```python
from build123d import *

# Parameters (mm, degrees)
BOSS_EXTRUDE1_DEPTH = 1.5
SKETCH3_W           = 6.5
SKETCH3_H           = 6.5
CUT_EXTRUDE1_DEPTH  = 2


with BuildPart() as part:
    # Sketch2 → Boss-Extrude1 (new body)
    with BuildSketch(Plane.XY):
        with BuildLine():
            Line((-7.517156851, 8.129598801), (22.482843149, 8.129598801))
            Line((22.482843149, 8.129598801), (22.482843149, -7.870401199))
            Line((22.482843149, -7.870401199), (12.482843149, -7.870401199))
            ThreePointArc((12.482843149, -7.870401199), (5.615628068, -3.288438903), (-2.517156851, -1.870401199))
            Line((-2.517156851, -1.870401199), (-7.517156851, -1.870401199))
            Line((-7.517156851, -1.870401199), (-7.517156851, 8.129598801))
        make_face()
    extrude(amount=BOSS_EXTRUDE1_DEPTH)

    # Sketch3 → Cut-Extrude1 (cut)
    with BuildSketch(Plane.XY.offset(1.5)):
        with Locations((16.232843149, -1.120401199)):
            Rectangle(SKETCH3_W, SKETCH3_H)
    extrude(amount=-CUT_EXTRUDE1_DEPTH, mode=Mode.SUBTRACT)


solid = part.part
```
Here's how the part is built. I have some questions about the finished solid (model axes, mm). A direction names the side the tool comes from. Give positions to 0.01 mm unless a question says otherwise; leave off trailing zeros. Write each loop counter-clockwise with the first axis right and the second up, starting at its lowest first coordinate (ties: lowest second). Pieces come first, ordered by that corner, then holes. Notation, with made-up numbers: M 31.5,80 L 72.5,80 A17 cw 72.5,100 Z; hole C 44,-8 d4. An arc over 180 degrees is marked long. Put each result on its own line as item: value. Start each with the question number.
Item 1: If we section it at A-A, the plane x = 16.25: Write out the boundary of the cut face in (y, z), then the cut area to 4 significant figures.
Item 2: If we section it at B-B, the plane y = 0.75: Write out the boundary of the cut face in (x, z), then the cut area to 4 significant figures.
Item 3: If we section it at C-C, the plane z = 0.7: Write out the boundary of the cut face in (x, y), then the cut area to 3 significant figures.
Item 4: If we section it at D-D, the plane x = -4.5: Write out the boundary of the cut face in (y, z).
Item 5: I need wall thicknesses on L1, parallel to Y at x = 16.75, z = 0.85; L2, parallel to X at y = -1.25, z = 0.6; L3, parallel to X at y = -3.5, z = 0.4. Which ranges of each line are inside material? Lowest first, please. Write a range as from..to.
Item 6: On a 3-axis mill with a long thin cutter (end or side, diameter ignored), from which of +Z, -Z, +X, -X, +Y, -Y can I reach the whole of each face in a straight line? I mean faces 4 (the flat face through (7, 8.13, 1)), 5 (the flat face through (19.483, -1, 1)). Say none if no direction works.
Item 7: Will this pin go through, and if not, where does the flat tip stop? pin 1 (0.8 mm diameter, centred on x = -6, z = 0.5, fed in from -Y).
Item 8: Thinking about a two-plate mould opening in Y: for faces 1 (the flat face through (-5, -1.87, 1)), 2 (the flat face through (16, 2.13, 1)), 3 (the flat face through (-7.517, 3, 1)), which applies, +Y half, -Y half, draft (parallel to the pull), parting line (faces both ways), or undercut?
Values:
1. outline: M -7.87,0 L -4.37,0 L -4.37,1.5 L -7.87,1.5 Z; M 2.13,0 L 8.13,0 L 8.13,1.5 L 2.13,1.5 Z
1. area: 14.25 mm²
2. outline: M -7.52,0 L 12.98,0 L 12.98,1.5 L -7.52,1.5 Z; M 19.48,0 L 22.48,0 L 22.48,1.5 L 19.48,1.5 Z
2. area: 35.25 mm²
3. outline: M -7.52,-1.87 L -2.52,-1.87 A20 cw 12.48,-7.87 L 22.48,-7.87 L 22.48,8.13 L -7.52,8.13 Z; hole M 12.98,-4.37 L 19.48,-4.37 L 19.48,2.13 L 12.98,2.13 Z
3. area: 344 mm²
4. outline: M -1.87,0 L 8.13,0 L 8.13,1.5 L -1.87,1.5 Z
5. L1: -7.87..-4.37, 2.13..8.13
5. L2: -7.52..12.98, 19.48..22.48
5. L3: 6.12..12.98, 19.48..22.48
6. face 4: +Z, -Z, +X, -X, +Y
6. face 5: +Z, -Z
7. pin 1: y = -1.87
8. face 1: -Y half
8. face 2: undercut
8. face 3: draft
